Solid Edge part; units mm, degrees
sketch "Sketch1" plane through (0, 0, 0) normal (0, 0, 1) x (1, 0, 0)
  circle A0 centre (0, 0) radius 9.525
extrude "Protrusion1" add sketch "Sketch1" along normal blind 7.9248
sketch "Sketch2" plane through (0, 0, 0) normal (0, 0, -1) x (0, 1, 0)
  circle A0 centre (0, 0) radius 6.35
extrude "Protrusion2" add sketch "Sketch2" along normal blind 12.7
sketch "Sketch3" plane through (0, 0, -12.7) normal (0, 0, -1) x (0, 1, 0)
  circle A0 centre (0, 0) radius 4.7625
extrude "Protrusion3" add sketch "Sketch3" along normal blind 15.875
sketch "Sketch4" plane through (0, 0, 7.9248) normal (0, 0, 1) x (0, 1, 0)
  line L0 (-3.175, 1.7461) -> (0, 3.8287)
  line L1 (-3.175, -2.051) -> (-3.175, 1.7461)
  line L2 (-3.175, -2.051) -> (0, -3.8287)
  line L3 (3.175, -2.051) -> (0, -3.8287)
  line L4 (3.175, -2.051) -> (3.175, 1.7461)
  line L5 (3.175, 1.7461) -> (0, 3.8287)
extrude "Cutout1" cut sketch "Sketch4" against normal blind 3.9624
chamfer "Chamfer1" distance 0.7874 angle 45 1 edges at (0, -4.7625, -28.575)
properties part number "55030020"
Verification items for the finished model (mm, model axes). A direction names the side the tool comes from. Give positions to 0.01 mm unless a question says otherwise; leave off trailing zeros. Loops run counter-clockwise (first coordinate to the right, second up) from the corner with the lowest first, then second, coordinate; pieces in that order, holes last. Notation, with made-up numbers: (49.5, -36.5) - (74.5, -36.5) arc R7 ccw to (74.5, -30.5) - close; hole circle Ø10 at (78.5, 25). An arc over 180 degrees is marked (long way). Write item = value, one per line. Start each with the question number.
Q1. Depth check by flat-ended pin: P1, Ø4, axis at x = -5.5, z = 2, coming from the -Y side; P2, Ø5, axis at x = -6.5, z = -5.5, coming from the -Y side; P3, Ø10, axis at x = 0, z = -21.5, coming from the -Y side. Enter the tip coordinate at first touch or a pass-through.
Q2. Cross-section at D-D, the plane y = -8. Enter the section's corners in (x, z), and give its area (3 significant figures).
Q3. Mould release check, pull along X, two halves, no side actions. Record for faces 1 (the face through (6.2, -1.38, -6.26)), 2 (the face through (2.927, -1.61, 5.971)), 3 (the face through (-1, 5, -12.7)): released by +X, released by -X, zero draft, split by the parting line, or undercut.
Q4. Thickness scan on line 1 (X direction, y = -8.25, z = 4.5); line 2 (Z direction, x = 4.25, y = 6.5); line 3 (Z direction, x = 6, y = -0.75). Record the ranges inside material, lowest first.
Q5. Tool access check on faces 4 (the face through (6.2, -2, 0)), 5 (the face through (0, 0, -28.575)), 6 (the face through (2.927, 1.61, 5.971)). Record the directions out of +Z, -Z, +X, -X, +Y, -Y that give a thin tool (end or side, any length) a straight path to the whole face; none if there is none.
Q6. Cross-section at B-B, the plane z = 3.5. Enter the section's corners in (x, y) (3 decimals), and give its area (3 significant figures).
Q7. Cross-section at C-C, the plane x = -5.5. Enter the section's corners in (y, z), and give its area (3 significant figures).
Answer key:
q1.P1 = -8.86
q1.P2 = -4.93
q1.P3 = -4.76
q2.outline = (-5.17, 0) - (5.17, 0) - (5.17, 7.92) - (-5.17, 7.92) - close
q2.area = 81.9 mm^2
q3.face_1 = split by the parting line
q3.face_2 = undercut
q3.face_3 = zero draft
q4.line_1 = -4.76 to 4.76
q4.line_2 = 0 to 7.92
q4.line_3 = -12.7 to 7.92
q5.face_4 = -Z
q5.face_5 = -Z, +X, -X, +Y, -Y
q5.face_6 = +Z
q6.outline = circle Ø19.05 at (0, 0)
q6.area = 285 mm^2
q7.outline = (-7.78, 0) - (-3.17, 0) - (-3.17, -12.7) - (3.17, -12.7) - (3.17, 0) - (7.78, 0) - (7.78, 7.92) - (-7.78, 7.92) - close
q7.area = 204 mm^2
